Build history of the part. All positions in model axes, mm. A direction names the side the tool comes from. Give positions to 0.01 mm unless a question says otherwise; leave off trailing zeros. Order: outer loops, then holes, each group sorted by start corner. A loop starts at its lowest first (then second) coordinate and runs counter-clockwise, first axis right, second up. Notation, with made-up numbers: (20, 79) - (73, 79) arc R19 ccw to (73, 98) - close; hole circle Ø6 at (64, 11.25). An arc over 180 degrees is marked (long way). Use a Markdown table: item, result. Add a question column.
(1) Slice it at A-A (y = 0). Write the cut outline in (x, z).
(2) Mould opens along X. For faces 1 (the face through (-8, 13, 48)), 2 (the face through (0, 4, 65)), 3 (the face through (0, 0, -12)) say: +X half, -X half, draft (parallel to the pull), parting line (faces both ways), or undercut.
(3) Slice it at C-C (z = 18). Write the cut outline in (x, y).
(4) Slice it at B-B (x = 0). Write the cut outline in (y, z).
(5) Flat gauge pins, fed straight in: pin 1 (8 mm diameter, centred on x = -7, z = 16, fed in from -Y) (3 decimals); pin 2 (3 mm diameter, centred on y = 13, z = 2.5, fed in from +X); pin 3 (2.5 mm diameter, centred on x = -0.5, z = 64.5, fed in from +Y). Where does each tip first touch, or does it go through?
(6) Which spindle directions (+Z, -Z, +X, -X, +Y, -Y) get a long thin tool onto all of the face, cutting with end or side? Do faces 4 (the face through (3.566, 16.059, -5.916)), 5 (the face through (0, 7, 71)), 6 (the face through (6.644, 14.437, 51.042)). Say none if no direction does.
(7) Wall check: line 1 (Z direction, x = 9, y = -5); line 2 (Z direction, x = 0, y = 1.5); line 3 (Y direction, x = 7, z = 50). Give the ranges that are in metal, low to high.
(8) Slice it at D-D (x = -5). Write the cut outline in (y, z), then the cut area to 3 significant figures.
Autodesk Inventor part; units mm, degrees
ref_plane "YZ Plane" through (0, 0, 0) normal (1, 0, 0) x (0, 1, 0)
ref_plane "XZ Plane" through (0, 0, 0) normal (0, 1, 0) x (-1, 0, 0)
ref_plane "XY Plane" through (0, 0, 0) normal (0, 0, 1) x (1, 0, 0)
sketch "Sketch1" plane through (0, 0, 0) normal (0, 0, 1) x (1, 0, 0)
  circle A0 centre (0, 0) radius 16.5
  dimension "d0" = 33
extrude "Extrusion1" add sketch "Sketch1" along normal blind 29
sketch "Sketch2" plane through (0, 0, 29) normal (0, 0, 1) x (1, 0, 0)
  circle A0 centre (0, 0) radius 18.5
  dimension "d3" = 37
extrude "Extrusion2" add sketch "Sketch2" along normal blind 24
sketch "Sketch3" plane through (0, 0, 53) normal (0, 0, 1) x (1, 0, 0)
  line L0 (0, 0) -> (0, 7)
  circle A0 centre (0, 7) radius 6
  dimension "d6" = 7
  dimension "d7" = 12
extrude "Extrusion3" add sketch "Sketch3" along normal blind 6
sketch "Sketch4" plane through (0, 7, 59) normal (0, 0, 1) x (1, 0, 0)
  circle A0 centre (0, 0) radius 6
  arc A1 (-1.199, 2.75) -> (1.199, 2.75) centre (0, 0) ccw
  line L0 (0, 0) -> (0, 2.75)
  line L1 (0, 2.75) -> (1.199, 2.75)
  line L2 (0, 2.75) -> (-1.199, 2.75)
  point P0 (0, -7)
  dimension "d10" = 6
  dimension "d11" = 2.75
extrude "Extrusion4" add sketch "Sketch4" along normal blind 12 contours L2 L1 A1
sketch "Sketch5" plane through (0, 0, 0) normal (0, 0, -1) x (-1, 0, 0)
  circle A0 centre (0, 0) radius 16.45
  dimension "d16" = 32.9
extrude "Extrusion5" add sketch "Sketch5" along normal blind 12
sketch "Sketch6" plane through (0, 0, 53) normal (0, 0, 1) x (1, 0, 0)
  circle A0 centre (0, 0) radius 18.5
  arc A1 (-3.1779, 12.0893) -> (3.1779, 12.0893) centre (0, 0) ccw
  circle A2 centre (0, 7) radius 6
  dimension "d17" = 25
extrude "Extrusion6" add sketch "Sketch6" along normal blind 1
sketch "Sketch8" plane through (0, 0, 54) normal (0, 0, 1) x (1, 0, 0)
  circle A0 centre (0, 0) radius 18.5
  arc A1 (-3.1779, 12.0893) -> (3.1779, 12.0893) centre (0, 0) ccw
  line L0 (12.5, 0) -> (18.5, 0)
  circle A2 centre (15.5, 0) radius 1.5
  circle A3 centre (7.75, 13.4234) radius 1.5
  circle A4 centre (-7.75, 13.4234) radius 1.5
  circle A5 centre (-15.5, 0) radius 1.5
  circle A6 centre (-7.75, -13.4234) radius 1.5
  circle A7 centre (7.75, -13.4234) radius 1.5
  arc A8 (-1.199, 9.75) -> (1.199, 9.75) centre (0, 7) ccw
  line L1 (-1.199, 9.75) -> (1.199, 9.75)
  circle A9 centre (0, 7) radius 6
  circle A10 centre (0, 7) radius 6
  line L2 (1.199, 9.75) -> (-1.199, 9.75)
  arc A11 (-1.199, 9.75) -> (1.199, 9.75) centre (0, 7) ccw
  dimension "d44" = 3
  dimension "d47" = 360
extrude "Extrusion7" cut sketch "Sketch8" against normal blind 6 contours A2 L0 | L0 A2 | A3 | A4 | A5 | A6 | A7
thread "Thread7"
thread "Thread8"
thread "Thread9"
thread "Thread10"
thread "Thread11"
thread "Thread12"
sketch "Sketch9" plane through (0, 7, 71) normal (0, 0, 1) x (1, 0, 0)
  line L0 (1.199, 2.75) -> (-1.199, 2.75)
  arc A0 (-1.199, 2.75) -> (1.199, 2.75) centre (0, 0) ccw
  circle A1 centre (0, -7) radius 18.5
  circle A2 centre (-7.75, -20.4234) radius 1.5
  line L1 (0, 0) -> (-7.75, -20.4234)
  circle A3 centre (0, -7) radius 16.5
  circle A4 centre (7.75, -20.4234) radius 1.5
  circle A5 centre (-7.75, 6.4234) radius 1.5
  line L2 (7.75, -20.4234) -> (-7.75, 6.4234)
  line L3 (0, -7) -> (-10.8253, -13.25)
  arc A6 (-3.1779, 5.0893) -> (3.1779, 5.0893) centre (0, -7) ccw
  line L4 (-16.8637, 0.607) -> (0, -7)
  line L5 (0, -7) -> (-16.8637, 0.607)
  line L6 (-16.8637, 0.607) -> (-26.1272, -19.9291)
  line L7 (-7.75, -20.4234) -> (-23.3448, -13.7609)
  line L8 (0, 0) -> (4.1821, 11.0211)
  line L9 (0, 0) -> (-13.8561, 5.2579)
  line L10 (-13.8561, 5.2579) -> (18.5, -7.0201)
  circle A7 centre (0, -7) radius 18.5
  line L11 (0, 0) -> (18.5, -7.0201)
sketch "Sketch10" plane through (0, 0, -12) normal (0, 0, -1) x (-1, 0, 0)
  circle A0 centre (0, 0) radius 16.5
  line L0 (0, 16.5) -> (0, -16.5)
  line L1 (-16.5, 0) -> (16.5, 0)
ref_plane "Work Plane1" through (16.5, 0, -12) normal (0, -1, 0) x (-1, 0, 0)
ref_plane "Work Plane2" through (0, 16.5, -12) normal (1, 0, 0) x (0, -1, 0)
properties part number "251RPM-Motor"
Solution:
| question | item | result |
|---|---|---|
| 1 | outline | (-18.5, 29) - (-16.5, 29) - (-16.5, 0) - (-16.45, 0) - (-16.45, -12) - (16.45, -12) - (16.45, 0) - (16.5, 0) - (16.5, 29) - (18.5, 29) - (18.5, 54) - (17, 54) - (17, 48) - (14, 48) - (14, 54) - (12.5, 54) - (12.5, 53) - (-12.5, 53) - (-12.5, 54) - (-14, 54) - (-14, 48) - (-17, 48) - (-17, 54) - (-18.5, 54) - close |
| 2 | face 1 | undercut |
| 2 | face 2 | parting line |
| 2 | face 3 | draft |
| 3 | outline | circle Ø33 at (0, 0) |
| 4 | outline | (-18.5, 29) - (-16.5, 29) - (-16.5, 0) - (-16.45, 0) - (-16.45, -12) - (16.45, -12) - (16.45, 0) - (16.5, 0) - (16.5, 29) - (18.5, 29) - (18.5, 54) - (13, 54) - (13, 59) - (9.75, 59) - (9.75, 71) - (4, 71) - (4, 59) - (1, 59) - (1, 53) - (-12.5, 53) - (-12.5, 54) - (-18.5, 54) - close |
| 5 | pin 1 | y = -16.225 |
| 5 | pin 2 | x = 11.83 |
| 5 | pin 3 | y = 9.75 |
| 6 | face 4 | -Z |
| 6 | face 5 | +Z, +X, -X, +Y, -Y |
| 6 | face 6 | +Z |
| 7 | line 1 | -12 to 53 |
| 7 | line 2 | -12 to 59 |
| 7 | line 3 | -17.12 to -14.72, -12.12 to 12.12, 14.72 to 17.12 |
| 8 | outline | (-17.81, 29) - (-15.72, 29) - (-15.72, 0) - (-15.67, 0) - (-15.67, -12) - (15.67, -12) - (15.67, 0) - (15.72, 0) - (15.72, 29) - (17.81, 29) - (17.81, 54) - (11.46, 54) - (11.46, 53) - (10.32, 53) - (10.32, 59) - (3.68, 59) - (3.68, 53) - (-11.46, 53) - (-11.46, 54) - (-17.81, 54) - close |
| 8 | area | 2,200 mm2 |
